Work out the finished part from the listing and answer in its coordinate system (mm). A direction names the side the tool comes from. Coordinates: 2 decimals unless noted, no trailing zeros. Order: outer loops, then holes, each group sorted by start corner. A loop starts at its lowest first (then second) coordinate and runs counter-clockwise, first axis right, second up. Notation, with made-up numbers: M 70,24 L 119,24 A9 cw 119,33 Z; hole C -6,36.5 d10. An arc over 180 degrees is marked long. Write item = value, one per line. Start each with the question number.
Q1. A tool of negligible diameter and unlimited length cuts with its end or side. For faces 1 (the cylindrical face through (10.19, 31.94, -4.47)), 2 (the cylindrical face through (-10.193, 29.009, -5.01)), 3 (the cylindrical face through (-10.95, 28.25, -5.15)), from which of +Z, -Z, +X, -X, +Y, -Y can it reach the whole face along a straight path? Write none if from no direction.
Q2. Determine the mould class of faces 4 (the cylindrical face through (-10.96, 32.7, -4.39)), 5 (the flat face through (0.158, 28.41, -3.115)), 6 (the cylindrical face through (10.96, 32.7, -4.39)), 7 (the flat face through (-0.14, 32, -4.46)) for opening direction X: released by +X, released by -X, zero draft, split by the parting line, or undercut.
Q3. Straight lines are drawn through the part: line 1 along X through (y, z) = (31, -4.35); line 2 along Y through (x, z) = (4, -5.8); line 3 along Y through (x, z) = (-9, -4.45). For each, find the intervals that lie inside material, in ascending order.
Q4. Find section A-A on x = -7.25. Give the vertices of the cut face in (y, z), and give its area (3 significant figures).
Q5. Each of these flat-tipped pins is pushed along its axis until it touches: P1, Ø3, axis at x = 1, y = 32, coming from the -Z side; P2, Ø1.5, axis at x = 7.5, z = -5, coming from the +Y side. Where does it stop, or does it pass through?
Q6. Find section B-B on y = 30.8. Give the vertices of the cut face in (x, z), and give its area (3 significant figures).
```python
from build123d import *

# Parameters (mm, degrees)
PAD003_DEPTH = 11.25
POCKET_DEPTH = 5
FILLET001_R  = 1


with BuildPart() as part:
    # Sketch → Pad003 (new body, symmetric)
    with BuildSketch(Plane.YZ):
        Polygon((27.6094120011, -3.2625768801), (32.625282988, -2.3400595397), (33.348826, -6.274076), (28.3329550131, -7.1965933403), align=None)
    extrude(amount=PAD003_DEPTH, both=True)

    # Sketch032 (on Face1 of Pad003) → Pocket (cut)
    with BuildSketch(Plane(origin=(0, 1.4837890217, -8.0675928562), x_dir=(0, -0.9835041151, -0.180885753), z_dir=(0, -0.180885753, 0.9835041151))):
        with BuildLine():
            Line((-30.463816642, 10.25), (-27.763816642, 10.25))
            ThreePointArc((-27.563816642, 10.05), (-27.6223952858, 10.1914213562), (-27.763816642, 10.25))
            Line((-27.563816642, 10.05), (-27.563816642, -10.05))
            ThreePointArc((-27.763816642, -10.25), (-27.6223952858, -10.1914213562), (-27.563816642, -10.05))
            Line((-27.763816642, -10.25), (-30.463816642, -10.25))
            ThreePointArc((-30.663816642, -10.05), (-30.6052379983, -10.1914213562), (-30.463816642, -10.25))
            Line((-30.663816642, -10.05), (-30.663816642, 10.05))
            ThreePointArc((-30.463816642, 10.25), (-30.6052379983, 10.1914213562), (-30.663816642, 10.05))
        make_face()
    extrude(amount=-POCKET_DEPTH, mode=Mode.SUBTRACT)

    # Fillet001
    fillet001_edges = [part.edges().sort_by_distance(p)[0] for p in [
        (11.25, 32.987054, -4.307068),
        (11.25, 27.971184, -5.229585),
        (-11.25, 32.987054, -4.307068),
        (-11.25, 27.971184, -5.229585),
    ]]
    fillet(fillet001_edges, radius=FILLET001_R)


solid = part.part
```
Findings below:
q1.face_1 = -Z
q1.face_2 = +Z
q1.face_3 = -Z, -X, -Y
q2.face_4 = released by -X
q2.face_5 = zero draft
q2.face_6 = released by +X
q2.face_7 = undercut
q3.line_1 = -11.25 to -10.25, 10.25 to 11.25
q3.line_2 = 28.08 to 29.09, 32.24 to 33.26
q3.line_3 = 27.83 to 28.84, 32 to 33.01
q4.outline = M 27.61,-3.26 L 28.33,-7.2 L 29.32,-7.02 L 28.59,-3.08 Z; M 31.64,-2.52 L 32.37,-6.45 L 33.35,-6.27 L 32.63,-2.34 Z
q4.area = 8.00 mm^2
q5.P1 = -6.45
q5.P2 = 33.25
q6.outline = M -11.25,-6.74 L -10.25,-6.74 L -10.25,-2.68 L -11.25,-2.68 Z; M 10.25,-6.74 L 11.25,-6.74 L 11.25,-2.68 L 10.25,-2.68 Z
q6.area = 8.13 mm^2
